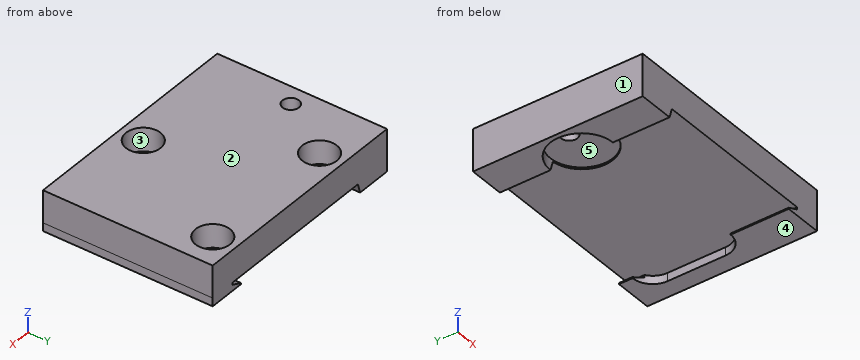
Autodesk Inventor part; units mm, degrees
ref_plane "YZ Plane" through (0, 0, 0) normal (1, 0, 0) x (0, 1, 0)
ref_plane "XZ Plane" through (0, 0, 0) normal (0, 1, 0) x (-1, 0, 0)
ref_plane "XY Plane" through (0, 0, 0) normal (0, 0, 1) x (1, 0, 0)
ref_plane "Work Plane1" through (52.5141, 202.7033, 6.4479) normal (0, 0, -1) x (0, 1, 0)
sketch "Sketch1" plane through (52.5141, 202.7033, 6.4479) normal (0, 0, -1) x (0, 1, 0)
  circle A0 centre (-59.8114, -30.5) radius 1.4 construction
  circle A1 centre (-38.8114, -18.3756) radius 1.4
  circle A2 centre (-38.8114, -42.6244) radius 1.4 construction
  circle A3 centre (41, 0) radius 1.65
  circle A4 centre (-9, 0) radius 1.65
  circle A5 centre (-9, 50) radius 1.65
  circle A6 centre (41, 50) radius 1.65
  circle A7 centre (16, 50) radius 1.65
  circle A8 centre (-9, 25) radius 1.65
  circle A9 centre (16, 0) radius 1.65
  circle A10 centre (41, 25) radius 1.65
  line L0 (80, 55) -> (-80, 55)
  line L1 (-80, 55) -> (-80, -55)
  line L2 (-80, -55) -> (80, -55)
  line L3 (80, -55) -> (80, 55)
  line L4 (-36.5, 0) -> (-36.5, -50)
  line L5 (-14, 0) -> (-36.5, 0)
  line L6 (-14, -5) -> (-14, 0)
  line L7 (72, -5) -> (-14, -5)
  line L8 (72, -50) -> (72, -5)
  line L9 (-36.5, -50) -> (72, -50)
  line L10 (-4, 45) -> (-4, 5)
  line L11 (36, 45) -> (-4, 45)
  line L12 (36, 5) -> (36, 45)
  line L13 (-4, 5) -> (36, 5)
  line L14 (-64.5989, -17.0433) -> (-64.5989, -57.0433) construction
  line L15 (-64.5989, -57.0433) -> (-34.5989, -57.0433) construction
  line L16 (-34.5989, -57.0433) -> (-34.5989, -17.0433) construction
  line L17 (-34.5989, -17.0433) -> (-64.5989, -17.0433) construction
  line L18 (-34.8114, -13.0433) -> (-63.8114, -13.0433)
  line L19 (-63.8114, -13.0433) -> (-63.8114, -52.6244)
  line L20 (-63.8114, -52.6244) -> (-34.8114, -52.6244)
  line L21 (-34.8114, -52.6244) -> (-34.8114, -13.0433)
  circle A11 centre (-59.8114, -30.5) radius 2.95
  circle A12 centre (-38.8114, -18.3756) radius 2.95
  circle A13 centre (-38.8114, -42.6244) radius 2.95 construction
  line L22 (-36.5, -35.1157) -> (-41.75, -35.1157) construction
  line L23 (-41.75, -35.1157) -> (-41.75, -38.5657) construction
  line L24 (-41.75, -38.5657) -> (-56.86, -38.5657) construction
  line L25 (-56.86, -38.5657) -> (-56.86, -35.1157) construction
  line L26 (-56.86, -35.1157) -> (-60.26, -35.1157) construction
  line L27 (-60.26, -35.1157) -> (-60.26, -52.0657) construction
  line L28 (-60.26, -52.0657) -> (-36.5, -52.0657) construction
  line L29 (-36.5, -52.0657) -> (-36.5, -35.1157) construction
  line L30 (-41.75, -28.3657) -> (-36.5, -28.3657) construction
  line L31 (-36.5, -28.3657) -> (-36.5, -25.0657) construction
  line L32 (-36.5, -25.0657) -> (-60.26, -25.0657) construction
  line L33 (-60.26, -25.0657) -> (-60.26, -28.3657) construction
  line L34 (-60.26, -28.3657) -> (-56.86, -28.3657) construction
  line L35 (-56.86, -28.3657) -> (-56.86, -27.0942) construction
  line L36 (-56.86, -27.0942) -> (-41.75, -27.0942) construction
  line L37 (-41.75, -27.0942) -> (-41.75, -28.3657) construction
  line L38 (-56.86, -35.1157) -> (-60.26, -35.1157) construction
  line L39 (-56.86, -38.5657) -> (-56.86, -35.1157) construction
  line L40 (-41.75, -38.5657) -> (-56.86, -38.5657) construction
  line L41 (-41.75, -35.1157) -> (-41.75, -38.5657) construction
  line L42 (-36.5, -35.1157) -> (-41.75, -35.1157) construction
  line L43 (-36.5, -35.05) -> (-36.5, -35.1157) construction
  line L44 (-36.5, -35.05) -> (-56.86, -35.05) construction
  line L45 (-36.5, -34.78) -> (-36.5, -35.05) construction
  line L46 (-36.5, -34.78) -> (-56.86, -34.78) construction
  line L47 (-36.5, -34.51) -> (-36.5, -34.78) construction
  line L48 (-36.5, -34.51) -> (-56.86, -34.51) construction
  line L49 (-36.5, -34.24) -> (-36.5, -34.51) construction
  line L50 (-36.5, -34.24) -> (-56.86, -34.24) construction
  line L51 (-36.5, -33.97) -> (-36.5, -34.24) construction
  line L52 (-36.5, -33.97) -> (-56.86, -33.97) construction
  line L53 (-36.5, -33.7) -> (-36.5, -33.97) construction
  line L54 (-36.5, -33.7) -> (-56.86, -33.7) construction
  line L55 (-36.5, -33.43) -> (-36.5, -33.7) construction
  line L56 (-36.5, -33.43) -> (-56.86, -33.43) construction
  line L57 (-36.5, -33.16) -> (-36.5, -33.43) construction
  line L58 (-36.5, -33.16) -> (-56.86, -33.16) construction
  line L59 (-36.5, -32.89) -> (-36.5, -33.16) construction
  line L60 (-36.5, -32.89) -> (-56.86, -32.89) construction
  line L61 (-36.5, -32.62) -> (-36.5, -32.89) construction
  line L62 (-36.5, -32.62) -> (-56.86, -32.62) construction
  line L63 (-36.5, -32.35) -> (-36.5, -32.62) construction
  line L64 (-36.5, -32.35) -> (-56.86, -32.35) construction
  line L65 (-36.5, -32.08) -> (-36.5, -32.35) construction
  line L66 (-36.5, -32.08) -> (-56.86, -32.08) construction
  line L67 (-36.5, -31.81) -> (-36.5, -32.08) construction
  line L68 (-36.5, -31.81) -> (-56.86, -31.81) construction
  line L69 (-36.5, -31.54) -> (-36.5, -31.81) construction
  line L70 (-36.5, -31.54) -> (-56.86, -31.54) construction
  line L71 (-36.5, -31.27) -> (-36.5, -31.54) construction
  line L72 (-36.5, -31.27) -> (-56.86, -31.27) construction
  line L73 (-36.5, -31) -> (-36.5, -31.27) construction
  line L74 (-36.5, -31) -> (-56.86, -31) construction
  line L75 (-36.5, -30.73) -> (-36.5, -31) construction
  line L76 (-36.5, -30.73) -> (-56.86, -30.73) construction
  line L77 (-36.5, -30.46) -> (-36.5, -30.73) construction
  line L78 (-36.5, -30.46) -> (-56.86, -30.46) construction
  line L79 (-36.5, -30.19) -> (-36.5, -30.46) construction
  line L80 (-36.5, -30.19) -> (-56.86, -30.19) construction
  line L81 (-36.5, -29.92) -> (-36.5, -30.19) construction
  line L82 (-36.5, -29.92) -> (-56.86, -29.92) construction
  line L83 (-36.5, -29.65) -> (-36.5, -29.92) construction
  line L84 (-36.5, -29.65) -> (-56.86, -29.65) construction
  line L85 (-36.5, -29.38) -> (-36.5, -29.65) construction
  line L86 (-36.5, -29.38) -> (-56.86, -29.38) construction
  line L87 (-36.5, -29.11) -> (-36.5, -29.38) construction
  line L88 (-36.5, -29.11) -> (-56.86, -29.11) construction
  line L89 (-36.5, -28.84) -> (-36.5, -29.11) construction
  line L90 (-36.5, -28.84) -> (-56.86, -28.84) construction
  line L91 (-36.5, -28.3657) -> (-36.5, -28.84) construction
  line L92 (-41.75, -28.3657) -> (-36.5, -28.3657) construction
  line L93 (-41.75, -27.0942) -> (-41.75, -28.3657) construction
  line L94 (-56.86, -27.0942) -> (-41.75, -27.0942) construction
  line L95 (-56.86, -28.3657) -> (-56.86, -27.0942) construction
  line L96 (-60.26, -28.3657) -> (-56.86, -28.3657) construction
  line L97 (-60.26, -35.1157) -> (-60.26, -28.3657) construction
  line L98 (-60.26, -25.0657) -> (-36.5, -25.0657) construction
  line L99 (-36.5, -25.0657) -> (-36.5, -52.0657) construction
  line L100 (-60.26, -52.0657) -> (-60.26, -25.0657) construction
  line L101 (-57.1632, -22.5233) -> (-33.4032, -22.5233) construction
  line L102 (-33.4032, -22.5233) -> (-33.4032, -49.5233) construction
  line L103 (-33.4032, -49.5233) -> (-57.1632, -49.5233) construction
  line L104 (-57.1632, -49.5233) -> (-57.1632, -22.5233) construction
  circle A14 centre (-38.8114, -42.6244) radius 2.95
  point P0 (-202.7033, -52.5141)
  point P1 (-56.7146, -27.9576)
  dimension "d0" = 4
  dimension "d2" = 4
  dimension "d3" = 4
  dimension "d4" = 5.9
  dimension "d5" = 5.9
  dimension "d6" = 5.9
  dimension "d10" = 10
  dimension "d35" = 24.2487
  dimension "d36" = 12.1244
extrude "Extrusion1" add sketch "Sketch1" along normal blind 4 contours L18 L21 L9 L4 A14 A12 | L4 A12 A14 L9 L21 L20 L19 L18
sketch "Sketch2" plane through (52.5141, 202.7033, 2.4479) normal (0, 0, -1) x (-1, 0, 0)
  circle A0 centre (42.6244, -38.8114) radius 2.95
  circle A1 centre (18.3756, -38.8114) radius 2.95
  circle A2 centre (30.5, -59.8114) radius 2.95
  line L0 (13.0433, -34.8114) -> (13.0433, -63.8114)
  line L1 (13.0433, -63.8114) -> (52.6244, -63.8114)
  line L2 (52.6244, -63.8114) -> (52.6244, -34.8114)
  line L3 (52.6244, -34.8114) -> (13.0433, -34.8114)
  point P0 (52.5141, -202.7033)
extrude "Extrusion2" add sketch "Sketch2" along normal blind 1.5 contours A0 | A1 | A2 | L3 L2 L1 L0
sketch "Sketch3" plane through (-0.1103, 138.8919, 6.4479) normal (0, -1, 0) x (1, 0, 0)
  line L0 (39.581, 0) -> (0, 0)
  line L1 (0, 0) -> (0, -5.5)
  line L2 (39.581, -5.5) -> (0, -5.5)
  line L3 (39.581, 0) -> (39.581, -5.5)
  line L4 (17.5087, -7.4479) -> (17.5087, -6.8479) construction
  line L5 (17.5087, -6.8479) -> (24.2587, -6.8479) construction
  line L6 (24.2587, -6.8479) -> (24.2587, -7.4479) construction
  line L7 (27.5587, -7.4479) -> (24.2587, -7.4479) construction
  line L8 (27.5587, -6.4479) -> (27.5587, -7.4479) construction
  line L9 (27.5587, -6.4479) -> (0.5587, -6.4479) construction
  line L10 (0.5587, -6.4479) -> (0.5587, -7.4479) construction
  line L11 (17.5087, -7.4479) -> (0.5587, -7.4479) construction
  line L12 (33.581, -5.5) -> (6.581, -5.5)
  line L13 (6.581, -5.5) -> (6.581, -6.5)
  line L14 (6.581, -6.5) -> (33.581, -6.5)
  line L15 (33.581, -6.5) -> (33.581, -5.5)
  line L16 (39.581, 0) -> (39.581, -5.5)
  line L17 (39.581, -5.5) -> (35.0732, -5.5)
  line L18 (35.0732, -5.5) -> (35.0732, -6.7)
  line L19 (35.0732, -6.7) -> (39.581, -6.7)
  line L20 (39.581, -6.7) -> (39.581, -5.5)
  line L21 (0, 0) -> (0, -5.5)
  line L22 (0, -5.5) -> (6.181, -5.5)
  line L23 (0, -7.2) -> (0, -5.5)
  line L24 (39.581, -6.7) -> (33.1536, -6.7)
  line L25 (33.1536, -6.7) -> (33.1536, -6.9)
  line L26 (33.1536, -6.9) -> (39.581, -6.9)
  line L27 (39.581, -6.9) -> (39.581, -6.7)
  line L28 (33.1536, -6.7) -> (35.0732, -5.8828)
  line L29 (0, -5.5) -> (39.581, -5.5)
  line L30 (6.6149, -5.5) -> (6.1022, -7.2)
  line L31 (6.1022, -7.2) -> (0, -7.2)
  dimension "d13" = 27
  dimension "d14" = 1
  dimension "d15" = 6
  dimension "d16" = 1.2
  dimension "d19" = 0.2
extrude "Extrusion3" add sketch "Sketch3" against normal up to surface (29 mm away) contours L20 L19 L18 L2 | L2 L13 L30 L31 L23 | L27 L26 L25 L24 L19 | L18 L24 L28 | L2 L30 L13
sketch "Sketch4" plane through (5.9919, 138.8919, -0.7521) normal (0, 0, -1) x (-1, 0, 0)
  line L0 (6.1022, 29) -> (0, 29)
  line L1 (0, 0) -> (0, 29)
  line L2 (6.1022, 0) -> (0, 0)
  line L3 (6.1022, 0) -> (6.1022, 29)
  circle A0 centre (0, 15.0183) radius 5.3352
  point P0 (5.9919, -138.8919)
extrude "Extrusion4" cut sketch "Sketch4" against normal blind 2 contours A0 L1 | L1 A0
sketch "Sketch5" plane through (52.5141, 202.7033, 0.9479) normal (0, 0, -1) x (-1, 0, 0)
  arc A0 (46.5221, -54.1283) -> (46.5221, -43.4579) centre (46.5221, -48.7931) ccw
  circle A1 centre (49.353, -48.7931) radius 1.4
  point P0 (52.5141, -202.7033)
  dimension "d30" = 2.8
extrude "Extrusion5" cut sketch "Sketch5" against normal through all
sketch "Sketch6" plane through (39.4707, 138.8919, -0.4521) normal (0, 0, -1) x (-1, 0, 0)
  line L0 (6.4274, 29) -> (0, 29)
  line L1 (0, 0) -> (0, 29)
  line L2 (6.4274, 0) -> (0, 0)
  line L3 (6.4274, 0) -> (6.4274, 29)
  arc A0 (33.4788, 9.6831) -> (33.4788, 20.3535) centre (33.4788, 15.0183) ccw
  line L4 (6.4274, 26.6901) -> (6.4274, 9.9295) construction
  line L5 (9.8619, 23.2557) -> (9.8619, 13.364)
  line L6 (2.993, 13.364) -> (2.993, 23.2557)
  arc A1 (9.8619, 23.2557) -> (2.993, 23.2557) centre (6.4274, 23.2557) ccw
  arc A2 (2.993, 13.364) -> (9.8619, 13.364) centre (6.4274, 13.364) ccw
  point P0 (39.4707, -138.8919)
  point P1 (6.4274, 18.3098)
extrude "Extrusion6" cut sketch "Sketch6" against normal up to surface (1.4 mm away) contours A1 L5 A2 L3 | L3 A2 L6 A1
equation "\"d31\" = d30"
properties part number "00_cellSTORM_v5_chiptray_old_0"
Geometry check sheet. Reference: the model listing, model coordinates, mm. Face numbers are marked on the shaded views. A direction names the side the tool comes from. Round coordinates to 2 decimals unless told otherwise and drop trailing zeros. Write each loop counter-clockwise with the first axis right and the second up, starting at its lowest first coordinate (ties: lowest second). Pieces come first, ordered by that corner, then holes. Notation, with made-up numbers: (-12, 9.5) -> (23, 9.5) arc R13 cw to (23, 14.5) -> close; hole circle Ø3 at (-32.75, 37.5). An arc over 180 degrees is marked (long way). One line per item, written item: value. Start each with the question number.
(1) Scan lines: line 1 (Y direction, x = 10, z = 3.5); line 2 (X direction, y = 161.25, z = 3.25); line 3 (X direction, y = 142.75, z = 4). Record each from-to range of solid material in increasing order. Write a range as [from, to].
(2) Go/stop test with flat-tipped pins: pin 1 Ø3 at (x, y) = (36, 158) entering from -Z; pin 2 Ø1.8 at (x, y) = (33, 165) entering from +Z; pin 3 Ø3 at (x, y) = (17, 156.5) entering from -Z. Record where each tip stops, or that it passes through.
(3) Access from +Z, -Z, +X, -X, +Y, -Y to the whole of each face (thin tool, end or side, straight path). Record for the marked faces 1, 2, 3, 4 and 5.
(4) Cross-section at C-C, the plane z = 4. Record the cut outline in (x, y).
(5) Cross-section at B-B, the plane x = 23. Record the cut outline in (y, z), and give its area (3 significant figures).
Answer:
1. line 1: [138.89, 160.94], [166.84, 167.89]
1. line 2: [-0.11, 8.58], [11.2, 32.83], [35.45, 39.47]
1. line 3: [-0.11, 19.07], [24.96, 39.47]
2. pin 1: z = -0.45
2. pin 2: z = 2.45
2. pin 3: z = 0.95
3. face 1: +Z, -Z, -X, +Y, -Y
3. face 2: +Z, +X, -X, +Y, -Y
3. face 3: +Z
3. face 4: -Z, +X, +Y, -Y
3. face 5: -Z
4. outline: (-0.11, 138.89) -> (39.47, 138.89) -> (39.47, 167.89) -> (-0.11, 167.89) -> close; hole circle Ø2.8 at (3.16, 153.91); hole circle Ø5.9 at (9.89, 163.89); hole circle Ø5.9 at (22.01, 142.89); hole circle Ø5.9 at (34.14, 163.89)
5. outline: (138.89, 0.95) -> (167.89, 0.95) -> (167.89, 6.45) -> (145.67, 6.45) -> (145.67, 2.45) -> (140.11, 2.45) -> (140.11, 6.45) -> (138.89, 6.45) -> close
5. area: 137 mm²
